For this review, use the dimensioned drawing (mm, ordinates from the lowest corner) and the shaded views. Give positions to 0.01 mm unless a question says otherwise; leave off trailing zeros. Write each loop counter-clockwise with the first axis right and the second up, starting at its lowest first coordinate (ties: lowest second). Pieces come first, ordered by that corner, then holes. Notation, with made-up numbers: M 56,-23 L 94,-23 A23 ccw 94,0 Z; hole C 75.5,47.25 d1. An arc over 180 degrees is marked long. Answer in a Markdown table with one row per item.
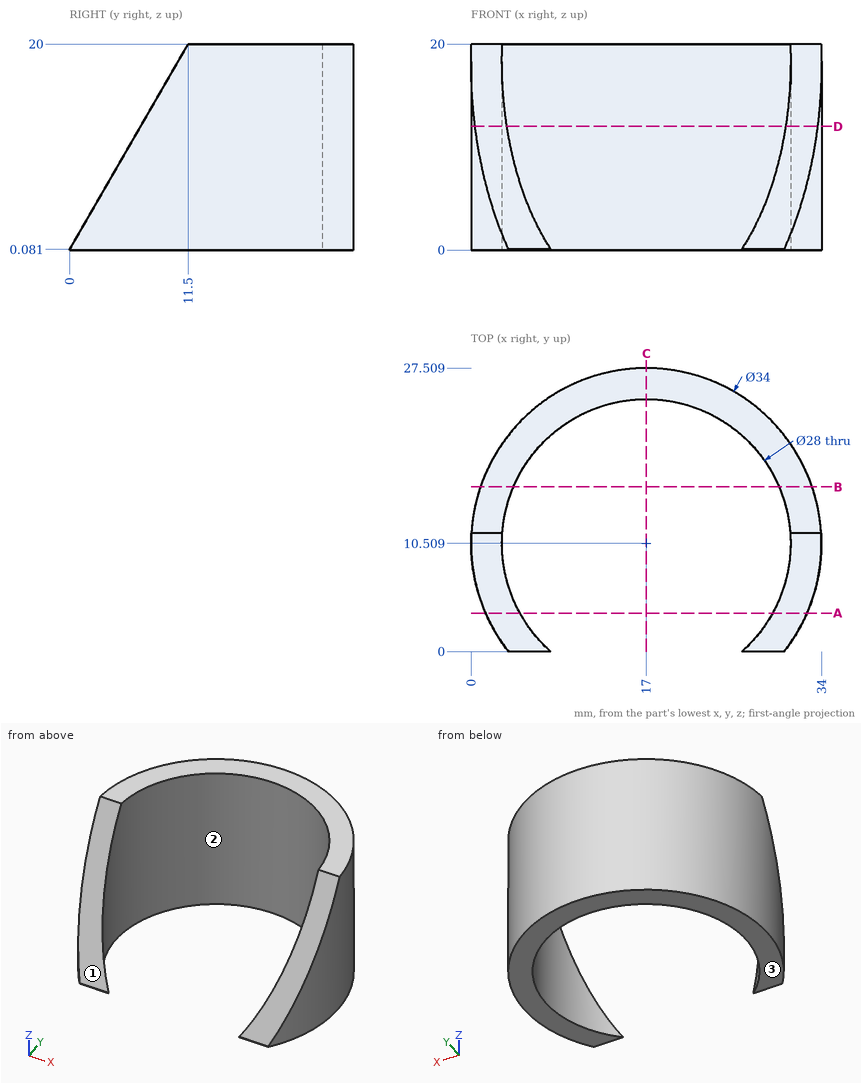
1) Add section A-A (y = 3.75). Write out the cut boundary in (x, z).
Geometry says:
| item | result |
|---|---|
| outline | M 1.4,0 L 4.74,0 L 4.74,6.58 L 1.4,6.58 Z; M 29.26,0 L 32.6,0 L 32.6,6.58 L 29.26,6.58 Z |
2) Add section B-B (y = 16). Write out the cut boundary in (x, z).
Geometry says:
| item | result |
|---|---|
| outline | M 0.91,0 L 4.12,0 L 4.12,20 L 0.91,20 Z; M 29.88,0 L 33.09,0 L 33.09,20 L 29.88,20 Z |
3) Insertion check: P1, Ø5, axis at x = 25.5, z = 16, coming from the +Y side (1 decimal); P2, Ø1, axis at y = 7, z = 5, coming from the +X side; P3, Ø6, axis at y = 7, z = 15.5, coming from the +X side. Each pin has a flat end and moves straight along its axis. Give the tip position at first contact, or say it passes through.
Geometry says:
| item | result |
|---|---|
| P1 | y = 26.4 |
| P2 | x = 33.73 |
| P3 | x = 33.99 |
4) The part is to be moulded in two halves that separate along Y. For the marked faces 1, 2 and 3, say which applies: released by +Y, released by -Y, zero draft, split by the parting line, or undercut.
Geometry says:
| item | result |
|---|---|
| face 1 | released by -Y |
| face 2 | undercut |
| face 3 | zero draft |
5) Add section D-D (z = 12). Write out the cut boundary in (x, y), and give its area (3 significant figures).
Geometry says:
| item | result |
|---|---|
| outline | M 0.39,6.88 L 3.48,6.88 A14 cw long 30.52,6.88 L 33.61,6.88 A17 ccw long Z |
| area | 168 mm^2 |
6) To check wall thickness, follow probe 1 along Y at (x, z) = (17, 15.5); probe 2 along X at (y, z) = (11.5, 4) (1 decimal); probe 3 along X at (y, z) = (8.25, 6.25). State the ranges of each line that lie inside material, in increasing order. Write a range as [from, to].
Geometry says:
| item | result |
|---|---|
| probe 1 | [24.51, 27.51] |
| probe 2 | [0, 3], [31, 34] |
| probe 3 | [0.15, 3.18], [30.82, 33.85] |
7) Add section C-C (x = 17). Write out the cut boundary in (y, z), and give its area (3 significant figures).
Geometry says:
| item | result |
|---|---|
| outline | M 24.51,0 L 27.51,0 L 27.51,20 L 24.51,20 Z |
| area | 60.0 mm^2 |
